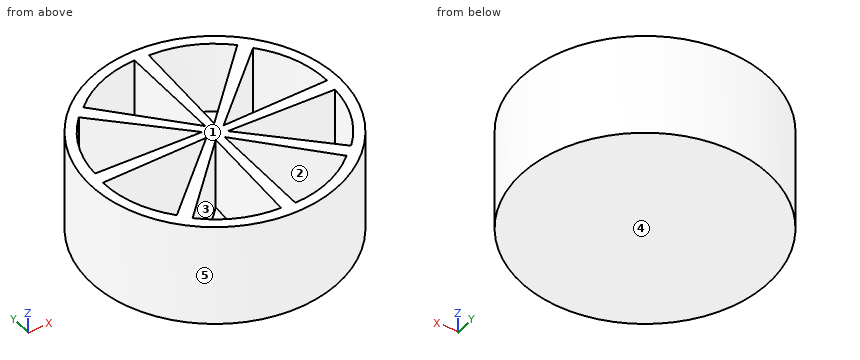
from build123d import *

# Parameters (mm, degrees)
CYLINDER001_W     = 10
CYLINDER001_H     = 12
CYLINDER001_ANGLE = 42
ARRAY_COUNT       = 8
CYLINDER_R        = 12
CYLINDER_DEPTH    = 10


with BuildPart() as array:
    # Cylinder001 → Cylinder001 (revolve)
    with BuildSketch(Plane(origin=(1, 0.25, 3), x_dir=(1, 0, 0), z_dir=(0, -1, 0))):
        with Locations((5, 6)):
            Rectangle(CYLINDER001_W, CYLINDER001_H)
    revolve(axis=Axis((1, 0.25, 3), (0, 0, 1)), revolution_arc=CYLINDER001_ANGLE)

    # Array: Array ×8 about axis
    array_axis = Axis((0, 0, 0), (0, 0, 1))


with BuildPart() as array_1:
    add(array.part)
    for i in range(1, ARRAY_COUNT):
        add(array.part.rotate(array_axis, i * 360 / ARRAY_COUNT))


with BuildPart() as cut:
    # Cylinder → Cylinder (new body)
    with BuildSketch(Plane.XY):
        Circle(CYLINDER_R)
    extrude(amount=CYLINDER_DEPTH)

    # Cut: cut Array
    add(array_1.part, mode=Mode.SUBTRACT)


solid = cut.part
Geometry: final body of the model. Coordinates: model frame, mm. Face numbers are marked on the shaded views. A direction names the side the tool comes from. Give positions to 0.01 mm unless a question says otherwise; leave off trailing zeros. Write each loop counter-clockwise with the first axis right and the second up, starting at its lowest first coordinate (ties: lowest second). Pieces come first, ordered by that corner, then holes.
(1) Cut plane B-B, the plane y = 6.25. Return loops of the section in (x, z).
(2) Cut plane D-D, the plane y = 1.5. Return loops of the section in (x, z), then the cut area to 3 significant figures.
(3) Cut plane A-A, the plane z = 4. Give the number of separate pieces and of enclosed holes in the cut face, then the cut area to 3 significant figures.
(4) Cut plane C-C, the plane x = -9.5. Return loops of the section in (y, z), then the cut area to 3 significant figures.
(5) Ray query, line 1 (X direction, y = 5.75, z = 5.75); line 2 (X direction, y = 2, z = 9.25); line 3 (Y direction, x = -8, z = 5). Return the intervals inside material, ascending.
(6) Mould query, pull axis X, two halves, no side actions, for the marked faces 3, 4 and 5. Classes: released by +X, released by -X, zero draft, split by the parting line, or undercut.
(7) Access query for the marked faces 1 and 2. Directions: +Z, -Z, +X, -X, +Y, -Y. A direction counts if a zero-diameter tool reaches every point of the face in a straight line with its end or side. Return the directions, or none.
(8) First-contact query: P1, Ø5.5, axis at x = 7, y = 4.5, coming from the +Z side; P2, Ø5.5, axis at y = -5.5, z = 8, coming from the +X side; P3, Ø2, axis at x = 8, y = -4.5, coming from the +Z side; P4, Ø3.5, axis at x = -3.5, z = 8, coming from the -Y side. Flat tips, straight axial feed; report the tip coordinate or a pass-through.
Values follow:
1. outline: (-10.24, 0) - (10.24, 0) - (10.24, 10) - (9, 10) - (9, 3) - (7.66, 3) - (7.66, 10) - (5.9, 10) - (5.9, 3) - (0.81, 3) - (0.81, 10) - (-0.25, 10) - (-0.25, 3) - (-4.98, 3) - (-4.98, 10) - (-6.6, 10) - (-6.6, 3) - (-9.09, 3) - (-9.09, 10) - (-10.24, 10) - close
2. outline: (-11.91, 0) - (11.91, 0) - (11.91, 10) - (10.92, 10) - (10.92, 3) - (2.39, 3) - (2.39, 10) - (1.15, 10) - (1.15, 3) - (0.56, 3) - (0.56, 10) - (-0.25, 10) - (-0.25, 3) - (-0.7, 3) - (-0.7, 10) - (-1.85, 10) - (-1.85, 3) - (-10.84, 3) - (-10.84, 10) - (-11.91, 10) - close
2. area: 108 mm2
3. separate pieces: 1
3. enclosed holes: 8
3. area: 159 mm2
4. outline: (-7.33, 0) - (7.33, 0) - (7.33, 10) - (5.61, 10) - (5.61, 3) - (0.98, 3) - (0.98, 10) - (-0.25, 10) - (-0.25, 3) - (-5.52, 3) - (-5.52, 10) - (-7.33, 10) - close
4. area: 77.4 mm2
5. line 1: x = -10.53 to -9.41, -6.1 to -4.53, -0.25 to 0.79, 5.4 to 7.11, 9.35 to 10.53
5. line 2: x = -11.83 to -10.78, -2.35 to -1.15, -0.25 to 0.59, 1.65 to 2.94, 10.85 to 11.83
5. line 3: y = -8.94 to -6.55, -0.25 to 0.9, 7.56 to 8.94
6. face 3: undercut
6. face 4: zero draft
6. face 5: split by the parting line
7. face 1: +Z, +X, -X, +Y, -Y
7. face 2: +Z
8. P1: stops at z = 10
8. P2: stops at x = 11.68
8. P3: stops at z = 3
8. P4: stops at y = -11.87
